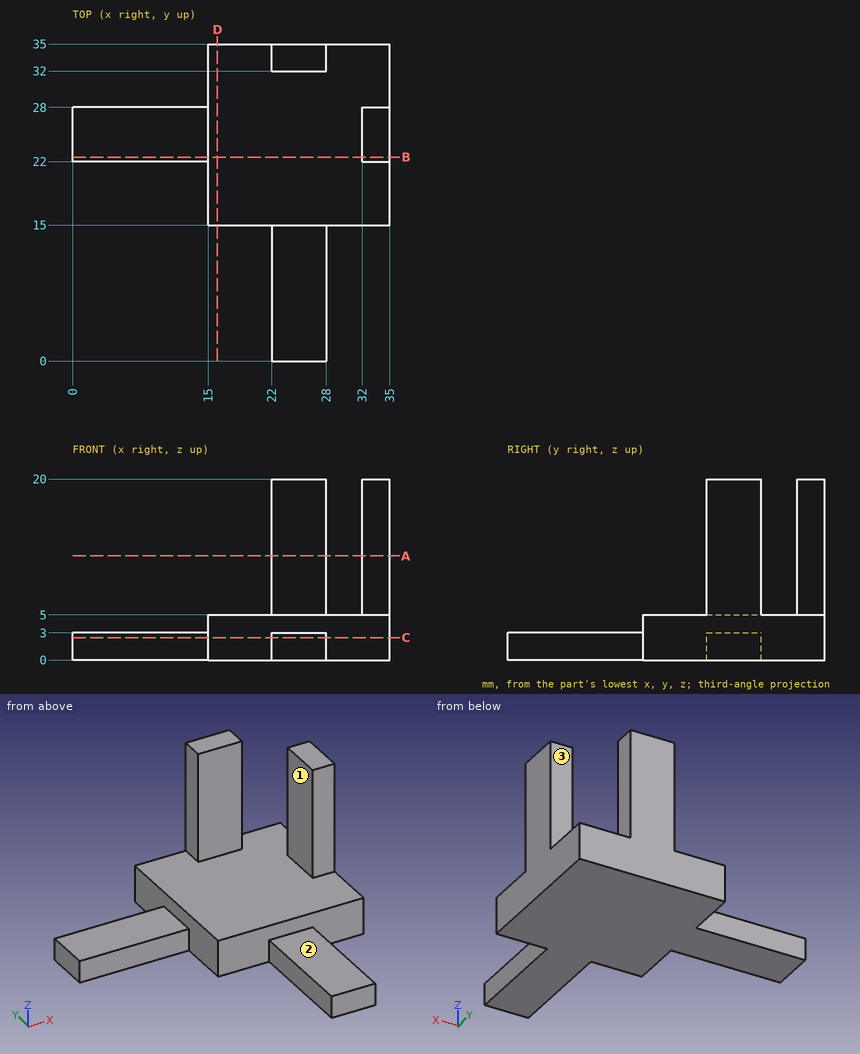
The figure shows three views and two pictorial views of one solid part (mm, origin at its lowest corner). Answer the questions. A direction names the side the tool comes from. Round coordinates to 2 decimals unless told otherwise and drop trailing zeros. Loops run counter-clockwise (first coordinate to the right, second up) from the corner with the lowest first, then second, coordinate; pieces in that order, holes last. Notation, with made-up numbers: M 21,20 L 28,20 A30 ccw 28,45 Z; hole C 66.5,7.5 d1. An arc over 180 degrees is marked long. Return JSON: item names as keys, results as strings.
Q1. Find the intervals of material crossed by line 1 along Z through (x, y) = (23.5, 26); line 2 along Z through (x, y) = (14, 26); line 3 along X through (y, z) = (27.5, 8.25), in increasing order. Write a range as from..to.
Results list:
{"line 1": "z = 0..5", "line 2": "z = 0..3", "line 3": "x = 32..35"}
Q2. Which of the six approach directions +Z, -Z, +X, -X, +Y, -Y give full straight-line access (tool end or side, diameter ignored) to the marked faces 1, 2 and 3?
Results list:
{"face 1": "+Z, -X, +Y, -Y", "face 2": "+Z, +X, -X, -Y", "face 3": "+Z, +X, -X, +Y"}
Q3. Find section A-A, the plane z = 11.5. Determine the outline of the cut face in (x, y), plus the area to 3 significant figures.
Results list:
{"outline": "M 22,32 L 28,32 L 28,35 L 22,35 Z; M 32,22 L 35,22 L 35,28 L 32,28 Z", "area": "36.0 mm2"}
Q4. Find section D-D, the plane x = 16. Determine the outline of the cut face in (y, z), plus the area to 3 significant figures.
Results list:
{"outline": "M 15,0 L 35,0 L 35,5 L 15,5 Z", "area": "100 mm2"}
Q5. Find section B-B, the plane y = 22.5. Determine the outline of the cut face in (x, z).
Results list:
{"outline": "M 0,0 L 35,0 L 35,20 L 32,20 L 32,5 L 15,5 L 15,3 L 0,3 Z"}
Q6. Find section C-C, the plane z = 2.5. Determine the outline of the cut face in (x, y), plus the area to 3 significant figures.
Results list:
{"outline": "M 0,22 L 15,22 L 15,15 L 22,15 L 22,0 L 28,0 L 28,15 L 35,15 L 35,35 L 15,35 L 15,28 L 0,28 Z", "area": "580 mm2"}
Q7. Each of these flat-tipped pins is pushed along its axis until it touches: pin 1 Ø4 at (x, z) = (21, 14) entering from -Y; pin 2 Ø0.9 at (x, z) = (10.5, 1) entering from +Y; pin 3 Ø10 at (x, y) = (11.5, 29.5) entering from +Z; pin 4 Ø1.5 at (x, z) = (21, 13) entering from +Y. Where does it stop, or does it pass through?
Results list:
{"pin 1": "stops at y = 32", "pin 2": "stops at y = 28", "pin 3": "stops at z = 5", "pin 4": "passes through"}
